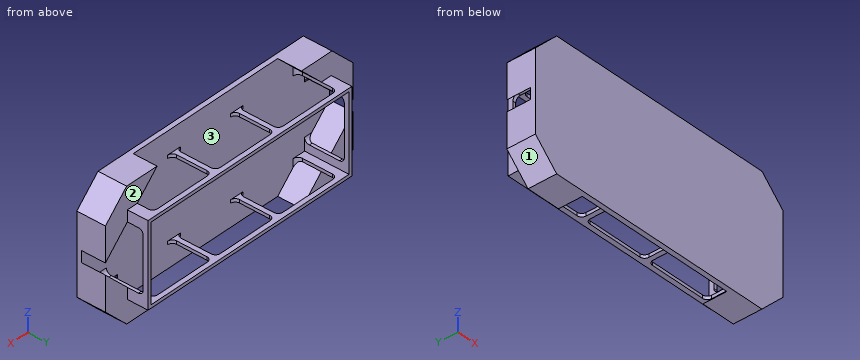
```python
from build123d import *

# Parameters (mm, degrees)
BASE_EXTRUSION_DEPTH         = 3
SKETCH_2_W                   = 144
SKETCH_2_H                   = 52
SKETCH_2_W_2                 = 140
SKETCH_2_H_2                 = 48
BATTERY_CASE_EXTRUSION_DEPTH = 28
BATTERY_CAGE_CUT_1_REACH     = 115.9
SKETCH_3_W                   = 41.333333333
SKETCH_3_H                   = 25
BATTERY_CAGE_CUT_2_REACH     = 169.336
SKETCH_4_W                   = 38
SKETCH_4_H                   = 25
EXTRUDE_1_DEPTH              = 15
FILLET_1_R                   = 3


with BuildPart() as part:
    # Эскиз1 → Base extrusion (new body)
    with BuildSketch(Plane(origin=(0, 0, 0), x_dir=(1, 0, 0), z_dir=(0, 1, 0))):
        Polygon((-87.5, 25), (-72.5, 40), (72.5, 40), (87.5, 25), (87.5, -25), (72.5, -40), (-72.5, -40), (-87.5, -25), align=None)
    extrude(amount=BASE_EXTRUSION_DEPTH)

    # Эскиз2 → Battery case extrusion (add)
    with BuildSketch(Plane(origin=(0, 3, 0), x_dir=(1, 0, 0), z_dir=(0, 1, 0))):
        Rectangle(SKETCH_2_W, SKETCH_2_H)
        Rectangle(SKETCH_2_W_2, SKETCH_2_H_2, mode=Mode.SUBTRACT)
    extrude(amount=BATTERY_CASE_EXTRUSION_DEPTH)

    # Battery cage cut 1: up to this face of the body (flat: up to its plane)
    battery_cage_cut_1_end = Plane(part.part.faces().sort_by_distance((0, 17, -26))[0])
    # Эскиз3 → Battery cage cut 1 (cut, up to the picked face)
    with BuildSketch(Plane.XY.offset(26), mode=Mode.PRIVATE) as battery_cage_cut_1_sk1:
        with Locations((-44.333333334, 15.5)):
            Rectangle(SKETCH_3_W, SKETCH_3_H)
    battery_cage_cut_1_tool1 = split(extrude(battery_cage_cut_1_sk1.sketch, amount=-BATTERY_CAGE_CUT_1_REACH, mode=Mode.PRIVATE), bisect_by=battery_cage_cut_1_end, keep=Keep.BOTH, mode=Mode.PRIVATE)
    # Эскиз3 → Battery cage cut 1 (cut, up to the picked face)
    with BuildSketch(Plane.XY.offset(26), mode=Mode.PRIVATE) as battery_cage_cut_1_sk2:
        with Locations((-0.003333334, 15.5)):
            Rectangle(SKETCH_3_W, SKETCH_3_H)
    battery_cage_cut_1_tool2 = split(extrude(battery_cage_cut_1_sk2.sketch, amount=-BATTERY_CAGE_CUT_1_REACH, mode=Mode.PRIVATE), bisect_by=battery_cage_cut_1_end, keep=Keep.BOTH, mode=Mode.PRIVATE)
    # Эскиз3 → Battery cage cut 1 (cut, up to the picked face)
    with BuildSketch(Plane.XY.offset(26), mode=Mode.PRIVATE) as battery_cage_cut_1_sk3:
        with Locations((44.326666667, 15.5)):
            Rectangle(SKETCH_3_W, SKETCH_3_H)
    battery_cage_cut_1_tool3 = split(extrude(battery_cage_cut_1_sk3.sketch, amount=-BATTERY_CAGE_CUT_1_REACH, mode=Mode.PRIVATE), bisect_by=battery_cage_cut_1_end, keep=Keep.BOTH, mode=Mode.PRIVATE)
    add(battery_cage_cut_1_tool1.solids().sort_by(Axis((-44.333333, 15.5, 26), (0, 0, -1)))[0], mode=Mode.SUBTRACT)
    add(battery_cage_cut_1_tool2.solids().sort_by(Axis((-0.003333, 15.5, 26), (0, 0, -1)))[0], mode=Mode.SUBTRACT)
    add(battery_cage_cut_1_tool3.solids().sort_by(Axis((44.326667, 15.5, 26), (0, 0, -1)))[0], mode=Mode.SUBTRACT)

    # Battery cage cut 2: up to this face of the body (flat: up to its plane)
    battery_cage_cut_2_end = Plane(part.part.faces().sort_by_distance((72, 17, 0))[0])
    # Эскиз4 → Battery cage cut 2 (cut, up to the picked face)
    with BuildSketch(Plane.ZY.offset(72), mode=Mode.PRIVATE) as battery_cage_cut_2_sk1:
        with Locations((0, 15.5)):
            Rectangle(SKETCH_4_W, SKETCH_4_H)
    battery_cage_cut_2_tool1 = split(extrude(battery_cage_cut_2_sk1.sketch, amount=-BATTERY_CAGE_CUT_2_REACH, mode=Mode.PRIVATE), bisect_by=battery_cage_cut_2_end, keep=Keep.BOTH, mode=Mode.PRIVATE)
    add(battery_cage_cut_2_tool1.solids().sort_by(Axis((-72, 15.5, 0), (1, 0, 0)))[0], mode=Mode.SUBTRACT)

    # Эскиз6 → Бобышка-Вытянуть1 (add)
    with BuildSketch(Plane(origin=(0, 3, 0), x_dir=(1, 0, 0), z_dir=(0, 1, 0))):
        Polygon((-87.5, 25), (-72.5, 40), (-51, 40), (-65, 26), (-72, 26), (-72, 19), (-87.5, 3.5), align=None)
        Polygon((65, 26), (72, 26), (72, 19), (87.5, 3.5), (87.5, 25), (72.5, 40), (51, 40), align=None)
        Polygon((-65, -26), (-72, -26), (-72, -19), (-87.5, -3.5), (-87.5, -25), (-72.5, -40), (-51, -40), align=None)
        Polygon((65, -26), (51, -40), (72.5, -40), (87.5, -25), (87.5, -3.5), (72, -19), (72, -26), align=None)
    extrude(amount=EXTRUDE_1_DEPTH)

    # Скругление1
    fillet_1_edges = [part.edges().sort_by_distance(p)[0] for p in [
        (71, 28, -19),
        (71, 3, 19),
        (71, 3, -19),
        (71, 28, 19),
        (-71, 3, -19),
        (-71, 28, -19),
        (-71, 28, 19),
        (-71, 3, 19),
        (-65, 28, -25),
        (-23.666666667, 3, -25),
        (-65, 3, -25),
        (-23.666666667, 28, -25),
        (-65, 3, 25),
        (-65, 28, 25),
        (-23.666666667, 28, 25),
        (-23.666666667, 3, 25),
        (-20.67, 28, -25),
        (20.663333333, 3, -25),
        (20.663333333, 28, -25),
        (-20.67, 3, -25),
        (-20.67, 28, 25),
        (20.663333333, 28, 25),
        (20.663333333, 3, 25),
        (-20.67, 3, 25),
        (23.66, 28, -25),
        (64.993333333, 3, -25),
        (64.993333333, 28, -25),
        (23.66, 3, -25),
        (23.66, 28, 25),
        (64.993333333, 28, 25),
        (64.993333333, 3, 25),
        (23.66, 3, 25),
    ]]
    fillet(fillet_1_edges, radius=FILLET_1_R)


solid = part.part
```
Work out the finished part from the listing and answer in its coordinate system (mm). Face numbers are marked on the shaded views. Round coordinates to 2 decimals unless told otherwise and drop trailing zeros. Loops run counter-clockwise (first coordinate to the right, second up) from the corner with the lowest first, then second, coordinate; pieces in that order, holes last. Notation, with made-up numbers: (-17, 71.25) -> (38, 71.25) arc R22 ccw to (38, 80.25) -> close; hole circle Ø7 at (-18, 7.25). An arc over 180 degrees is marked (long way). Write each question's results on one line, items separated by ' | '. Start each with the question number.
1. Section C-C (z = -32) is taken. Determine the outline of the cut face in (x, y).
2. Section D-D (z = -14) is taken. Determine the outline of the cut face in (x, y), plus the area to 3 significant figures.
3. Section A-A (z = 8) is taken. Determine the outline of the cut face in (x, y).
4. Section B-B (x = 38.5) is taken. Determine the outline of the cut face in (y, z), plus the area to 3 significant figures.
5. For a pull along Z with two mould halves and no side action, classify the marked faces 1, 2 and 3 as +Z half, -Z half, draft (parallel to the pull), parting line (faces both ways), or undercut.
6. Find the intervals of material crossed by probe 1 along X at (y, z) = (11, 25.5); probe 2 along X at (y, z) = (16.5, -19.5); probe 3 along X at (y, z) = (27, -23), in increasing order. Write a range as from..to.
7. Given pin 1 Ø1.5 at (x, z) = (69.5, 12) entering from +Y; pin 2 Ø8 at (x, y) = (17.5, 14.5) entering from -Z; pin 3 Ø10.5 at (y, z) = (27.5, 11) entering from -X; pin 4 Ø14 at (x, y) = (29.5, 19.5) entering from +Z, each flat-ended and moving along its own axis, determine where each tip first touches the part or whether it passes through.
Evaluation:
1) outline: (-80.5, 0) -> (80.5, 0) -> (80.5, 18) -> (59, 18) -> (59, 3) -> (-59, 3) -> (-59, 18) -> (-80.5, 18) -> close
2) outline: (-87.5, 0) -> (87.5, 0) -> (87.5, 18) -> (77, 18) -> (77, 3) -> (-77, 3) -> (-77, 18) -> (-87.5, 18) -> close; (-72, 28) -> (-70, 28) -> (-70, 31) -> (-72, 31) -> close; (70, 28) -> (72, 28) -> (72, 31) -> (70, 31) -> close | area: 852 mm2
3) outline: (-87.5, 0) -> (87.5, 0) -> (87.5, 18) -> (83, 18) -> (83, 3) -> (-83, 3) -> (-83, 18) -> (-87.5, 18) -> close; (-72, 28) -> (-70, 28) -> (-70, 31) -> (-72, 31) -> close; (70, 28) -> (72, 28) -> (72, 31) -> (70, 31) -> close
4) outline: (0, -40) -> (3, -40) -> (3, 40) -> (0, 40) -> close; (28, -26) -> (31, -26) -> (31, -24) -> (28, -24) -> close; (28, 24) -> (31, 24) -> (31, 26) -> (28, 26) -> close | area: 252 mm2
5) face 1: -Z half | face 2: draft | face 3: undercut
6) probe 1: x = -87..-65, -23.67..-20.67, 20.66..23.66, 64.99..87 | probe 2: x = -87.5..-70, 70..87.5 | probe 3: x = -72..-70, 70..72
7) pin 1: stops at y = 31 | pin 2: stops at z = -26 | pin 3: stops at x = -72 | pin 4: stops at z = 26
